Geometry check sheet. Reference: the model listing, model coordinates, mm. Coordinates: 2 decimals unless noted, no trailing zeros. Write each loop counter-clockwise with the first axis right and the second up, starting at its lowest first coordinate (ties: lowest second). Pieces come first, ordered by that corner, then holes. Notation, with made-up numbers: M 28.5,28 L 84.5,28 A10 ccw 84.5,44 Z; hole C -39,77.25 d11. An arc over 180 degrees is marked long. Write each question's results on one line, items separated by ' | '.
```python
from build123d import *

# Parameters (mm, degrees)
F3_DEPTH = 157.4
F4_DEPTH = 5
F6_DEPTH = 100


with BuildPart() as f3:
    # F2 (on offset) → F3 (new body)
    with BuildSketch(Plane.XZ.offset(76.2)):
        with BuildLine():
            ThreePointArc((15.32, 3.6), (16.644922, 2.012461), (17.12, 0))
            Line((17.12, 0), (20.12, 0))
            Line((20.12, 0), (15.32, 3.6))
        make_face()
        with BuildLine():
            ThreePointArc((-17.12, 0), (-16.644922, 2.012461), (-15.32, 3.6))
            Line((-15.32, 3.6), (-20.12, 0))
            Line((-20.12, 0), (-17.12, 0))
        make_face()
        with BuildLine():
            ThreePointArc((-4.5, 0), (-3.181981, 3.181981), (0, 4.5))
            Line((0, 4.5), (-12.62, 4.5))
            ThreePointArc((-12.62, 4.5), (-9.438019, 3.181981), (-8.12, 0))
            Line((-8.12, 0), (-4.5, 0))
        make_face()
        with BuildLine():
            ThreePointArc((0, 4.5), (3.181981, 3.181981), (4.5, 0))
            Line((4.5, 0), (8.12, 0))
            ThreePointArc((8.12, 0), (9.438019, 3.181981), (12.62, 4.5))
            Line((12.62, 4.5), (0, 4.5))
        make_face()
        with BuildLine():
            ThreePointArc((15.32, 3.6), (14.043025, 4.269075), (12.62, 4.5))
            Line((12.62, 4.5), (12.62, 0))
            Line((12.62, 0), (15.32, 3.6))
        make_face()
        with BuildLine():
            Line((0, 0), (4.5, 0))
            ThreePointArc((4.5, 0), (3.181981, 3.181981), (0, 4.5))
            Line((0, 4.5), (0, 0))
        make_face()
        with BuildLine():
            Line((0, 0), (0, 4.5))
            ThreePointArc((0, 4.5), (-3.181981, 3.181981), (-4.5, 0))
            Line((-4.5, 0), (0, 0))
        make_face()
        with BuildLine():
            Line((12.62, 0), (17.12, 0))
            ThreePointArc((17.12, 0), (16.644922, 2.012461), (15.32, 3.6))
            Line((15.32, 3.6), (12.62, 0))
        make_face()
        with BuildLine():
            ThreePointArc((12.62, 4.5), (9.438019, 3.181981), (8.12, 0))
            Line((8.12, 0), (12.62, 0))
            Line((12.62, 0), (12.62, 4.5))
        make_face()
        with BuildLine():
            Line((-12.62, 0), (-12.62, 4.5))
            ThreePointArc((-12.62, 4.5), (-14.043025, 4.269075), (-15.32, 3.6))
            ThreePointArc((-15.32, 3.6), (-16.644922, 2.012461), (-17.12, 0))
            Line((-17.12, 0), (-12.62, 0))
        make_face()
        with BuildLine():
            ThreePointArc((-8.12, 0), (-9.438019, 3.181981), (-12.62, 4.5))
            Line((-12.62, 4.5), (-12.62, 0))
            Line((-12.62, 0), (-8.12, 0))
        make_face()
    extrude(amount=-F3_DEPTH)

    # F3_face (on face) → F4 (join)
    with BuildSketch(Plane(origin=(0, -76.2, 2.111862), x_dir=(1, 0, 0), z_dir=(0, -1, 0))):
        with BuildLine():
            ThreePointArc((15.32, 1.488138), (14.043025, 2.157213), (12.62, 2.388138))
            Line((12.62, 2.388138), (-12.62, 2.388138))
            ThreePointArc((-12.62, 2.388138), (-14.043025, 2.157213), (-15.32, 1.488138))
            Line((-15.32, 1.488138), (-20.12, -2.111862))
            Line((-20.12, -2.111862), (20.12, -2.111862))
            Line((20.12, -2.111862), (15.32, 1.488138))
        make_face()
    extrude(amount=F4_DEPTH)

    # F5 (on Right) → F6 (cut, symmetric)
    with BuildSketch(Plane.YZ):
        Polygon((-81.2, 4.5), (-81.2, 0), (-76.2, 4.5), align=None)
    extrude(amount=F6_DEPTH, both=True, mode=Mode.SUBTRACT)


solid = f3.part
```
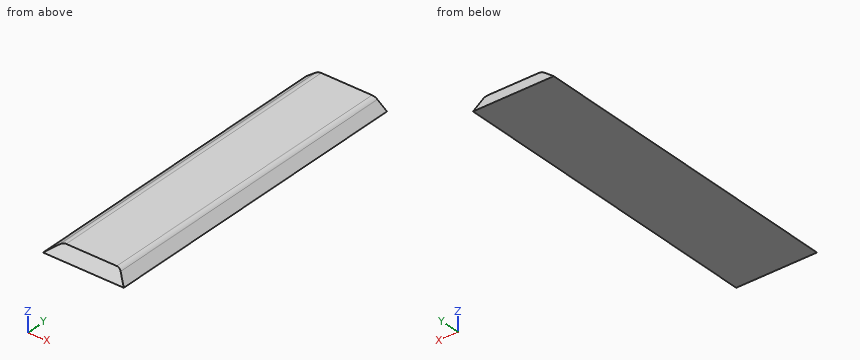
Q1. Sectioned sample at B-B on x = 5.5. Record the cut outline in (y, z), and give its area (3 significant figures).
Geometry check:
outline: M -81.2,0 L 81.2,0 L 81.2,4.5 L -76.2,4.5 Z | area: 720 mm2
Q2. Depth check by flat-ended pin: P1, Ø2, axis at y = 32, z = 3, coming from the +X side; P2, Ø1, axis at y = -10.5, z = 3.5, coming from the -X side; P3, Ø1, axis at y = -43, z = 2.5, coming from the -X side. Enter the tip coordinate at first touch or a pass-through.
Geometry check:
P1: stops at x = 17.45 | P2: stops at x = -16.12 | P3: stops at x = -17.45
Q3. Sectioned sample at A-A on y = -13.5. Record the cut outline in (x, z), and give its area (3 significant figures).
Geometry check:
outline: M -20.12,0 L 20.12,0 L 15.32,3.6 A4.5 ccw 12.62,4.5 L -12.62,4.5 A4.5 ccw -15.32,3.6 Z | area: 154 mm2
Q4. Scan lines: probe 1 along X at (y, z) = (-61.5, 2.6); probe 2 along X at (y, z) = (73, 4.1); probe 3 along Y at (x, z) = (-7.5, 3.7). Record each from-to range of solid material in increasing order.
Geometry check:
probe 1: x = -16.65 to 16.65 | probe 2: x = -14.47 to 14.47 | probe 3: y = -77.09 to 81.2
Q5. Sectioned sample at C-C on z = 2.6. Record the cut outline in (x, y), and give its area (3 significant figures).
Geometry check:
outline: M -16.65,-78.31 L 16.65,-78.31 L 16.65,81.2 L -16.65,81.2 Z | area: 5,310 mm2
